Verification items for the finished model (mm, model axes). A direction names the side the tool comes from. Give positions to 0.01 mm unless a question says otherwise; leave off trailing zeros. Write each loop counter-clockwise with the first axis right and the second up, starting at its lowest first coordinate (ties: lowest second). Pieces come first, ordered by that corner, then holes. Notation, with made-up numbers: (30.5, -31.5) -> (71.5, -31.5) arc R12 cw to (71.5, -9.5) -> close; hole circle Ø7 at (14, 78). An arc over 180 degrees is marked (long way). Use CSV: the item, a comma, the result in double quotes. Start each with the question number.
```python
from build123d import *

# Parameters (mm, degrees)
PAD_DEPTH    = 3.2
SKETCH001_R  = 1.19
POCKET_DEPTH = 3.201


with BuildPart() as part:
    # Sketch → Pad (new body)
    with BuildSketch(Plane.XZ):
        with BuildLine():
            Line((60, 0), (0, 0))
            Line((0, 0), (0, 36.25))
            ThreePointArc((6.5, 42.75), (1.903806, 40.846194), (0, 36.25))
            Line((6.5, 42.75), (11.5, 42.75))
            ThreePointArc((11.5, 42.75), (16.096194, 44.653806), (18, 49.25))
            Line((18, 49.25), (18, 87.75))
            ThreePointArc((21, 90.75), (18.87868, 89.87132), (18, 87.75))
            Line((21, 90.75), (57, 90.75))
            ThreePointArc((60, 87.75), (59.12132, 89.87132), (57, 90.75))
            Line((60, 87.75), (60, 0))
        make_face()
    extrude(amount=PAD_DEPTH)

    # Sketch001 (on Face12 of Pad) → Pocket (cut, through all)
    with BuildSketch(Plane.XZ.offset(3.2)):
        with Locations((19.19, 39.94)):
            Circle(SKETCH001_R)
        with Locations((2.69, 29.07)):
            Circle(SKETCH001_R)
        with Locations((2.69, 4.19)):
            Circle(SKETCH001_R)
    extrude(amount=-POCKET_DEPTH, mode=Mode.SUBTRACT)


solid = part.part
```
(1) Draft check along X on faces 1 (the face through (2.54, -1.62, 5.37)), 2 (the face through (1.955, -1.578, 40.896)), 3 (the face through (2.54, -1.62, 30.25)), 4 (the face through (37, 0, 46)). Enter one of: released by +X, released by -X, zero draft, split by the parting line, or undercut.
(2) Go/stop test with flat-tipped pins: pin 1 (1.6 mm diameter, centred on y = -2, z = 67, fed in from -X); pin 2 (1.5 mm diameter, centred on x = 35.5, y = -2.5, fed in from -Z). Record where each tip stops, or that it passes through.
(3) Section check C-C on y = -1.45. Record the cut outline in (x, z).
(4) Set-up check for faces 5 (the face through (18, -2, 68)), 6 (the face through (37, -3.2, 46)): record each of +Z, -Z, +X, -X, +Y, -Y from which the full face is reachable in a straight line by a thin tool's end or side.
(5) Section check D-D on x = 19.19. Record the cut outline in (y, z), then the cut area to 3 significant figures.
(6) Thickness scan on line 1 (Z direction, x = 2.69, y = -1.7); line 2 (X direction, y = -0.5, z = 69); line 3 (X direction, y = -1.25, z = 5). Record the ranges inside material, lowest first. Write a range as from..to.
(7) Section check A-A on z = 29.07. Record the cut outline in (x, y).
(8) Section check B-B on x = 2.69. Record the cut outline in (y, z), then the cut area to 3 significant figures.
Data:
1,face 1,"undercut"
1,face 2,"released by -X"
1,face 3,"undercut"
1,face 4,"zero draft"
2,pin 1,"stops at x = 18"
2,pin 2,"stops at z = 0"
3,outline,"(0, 0) -> (60, 0) -> (60, 87.75) arc R3 ccw to (57, 90.75) -> (21, 90.75) arc R3 ccw to (18, 87.75) -> (18, 49.25) arc R6.5 cw to (11.5, 42.75) -> (6.5, 42.75) arc R6.5 ccw to (0, 36.25) -> close; hole circle Ø2.38 at (2.69, 4.19); hole circle Ø2.38 at (2.69, 29.07); hole circle Ø2.38 at (19.19, 39.94)"
4,face 5,"+Z, -X, +Y, -Y"
4,face 6,"+Z, -Z, +X, -X, -Y"
5,outline,"(-3.2, 0) -> (0, 0) -> (0, 38.75) -> (-3.2, 38.75) -> close; (-3.2, 41.13) -> (0, 41.13) -> (0, 90.14) -> (-3.2, 90.14) -> close"
5,area,"281 mm2"
6,line 1,"z = 0..3, 5.38..27.88, 30.26..41.52"
6,line 2,"x = 18..60"
6,line 3,"x = 0..1.82, 3.56..60"
7,outline,"(0, -3.2) -> (1.5, -3.2) -> (1.5, 0) -> (0, 0) -> close; (3.88, -3.2) -> (60, -3.2) -> (60, 0) -> (3.88, 0) -> close"
8,outline,"(-3.2, 0) -> (0, 0) -> (0, 3) -> (-3.2, 3) -> close; (-3.2, 5.38) -> (0, 5.38) -> (0, 27.88) -> (-3.2, 27.88) -> close; (-3.2, 30.26) -> (0, 30.26) -> (0, 41.52) -> (-3.2, 41.52) -> close"
8,area,"118 mm2"
